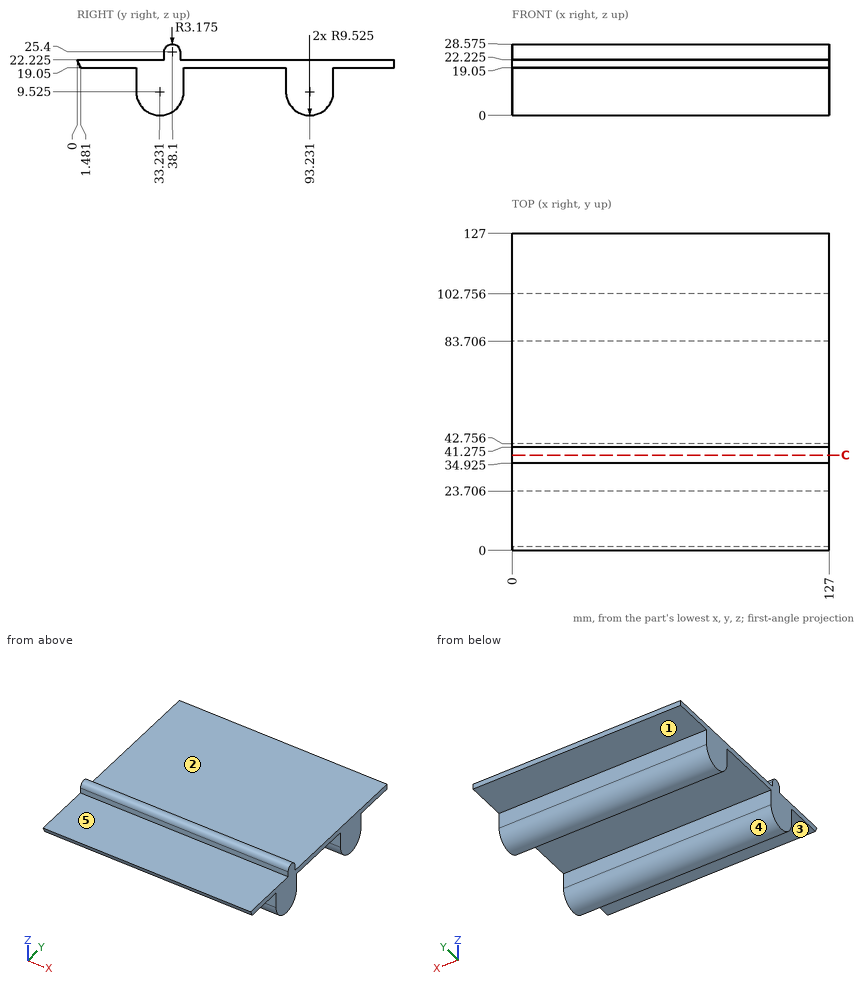
Here's the drawing with two shaded views (mm, measured from the low corner). I have some questions. A direction names the side the tool comes from. Round coordinates to 2 decimals unless told otherwise and drop trailing zeros. Loops run counter-clockwise (first coordinate to the right, second up) from the corner with the lowest first, then second, coordinate; pieces in that order, holes last.
Item 1: Will these pins go through, and if not, where does the flat tip stop? pin 1 Ø12 at (x, y) = (78.5, 112.5) entering from -Z; pin 2 Ø1 at (x, z) = (44.5, 23.5) entering from -Y (3 decimals); pin 3 Ø4 at (x, z) = (93, 10.5) entering from +Y.
Item 2: Please list where these lines run through material, in increasing order: L1, parallel to Y at x = 34, z = 14 (1 decimal); L2, parallel to Y at x = 86.5, z = 24 (1 decimal); L3, parallel to Y at x = 19, z = 3.5 (1 decimal).
Item 3: Which directions (+Z, -Z, +X, -X, +Y, -Y) give clear straight access to the entire face, cutting with the end or side of a thin tool? Please do the marked faces 1, 2 and 3.
Item 4: If we mould it in two halves opening along Y, with no side actions, what happens to the marked faces 4 and 5? For each: +Y half, -Y half, draft (parallel to the pull), parting line (faces both ways), or undercut.
Item 5: Suppose I cut it at C-C, the plane y = 38.1. Write out the boundary of the cut face in (x, z) (1 decimal), then the cut area to 3 significant figures.
Reported:
1. pin 1: stops at z = 19.05
1. pin 2: stops at y = 34.925
1. pin 3: stops at y = 102.76
2. L1: y = 23.7 to 42.8, 83.7 to 102.8
2. L2: y = 34.9 to 41.3
2. L3: y = 25.9 to 40.6, 85.9 to 100.6
3. face 1: -Z, +X, -X, +Y
3. face 2: +Z, +X, -X, +Y
3. face 3: -Z, +X, -X, -Y
4. face 4: undercut
4. face 5: draft
5. outline: (0, 1.3) - (127, 1.3) - (127, 28.6) - (0, 28.6) - close
5. area: 3,460 mm2
